Source: three-view drawing plus pictorial views. Frame: mm from the lowest corner of the part. A direction names the side the tool comes from. Give positions to 0.01 mm unless a question says otherwise; leave off trailing zeros. Loops run counter-clockwise (first coordinate to the right, second up) from the corner with the lowest first, then second, coordinate; pieces in that order, holes last. Notation, with made-up numbers: M 23,52.25 L 40,52.25 A17 cw 40,66.25 Z; hole C -16,72.25 d1. An arc over 180 degrees is marked long. Write item = value, one per line.
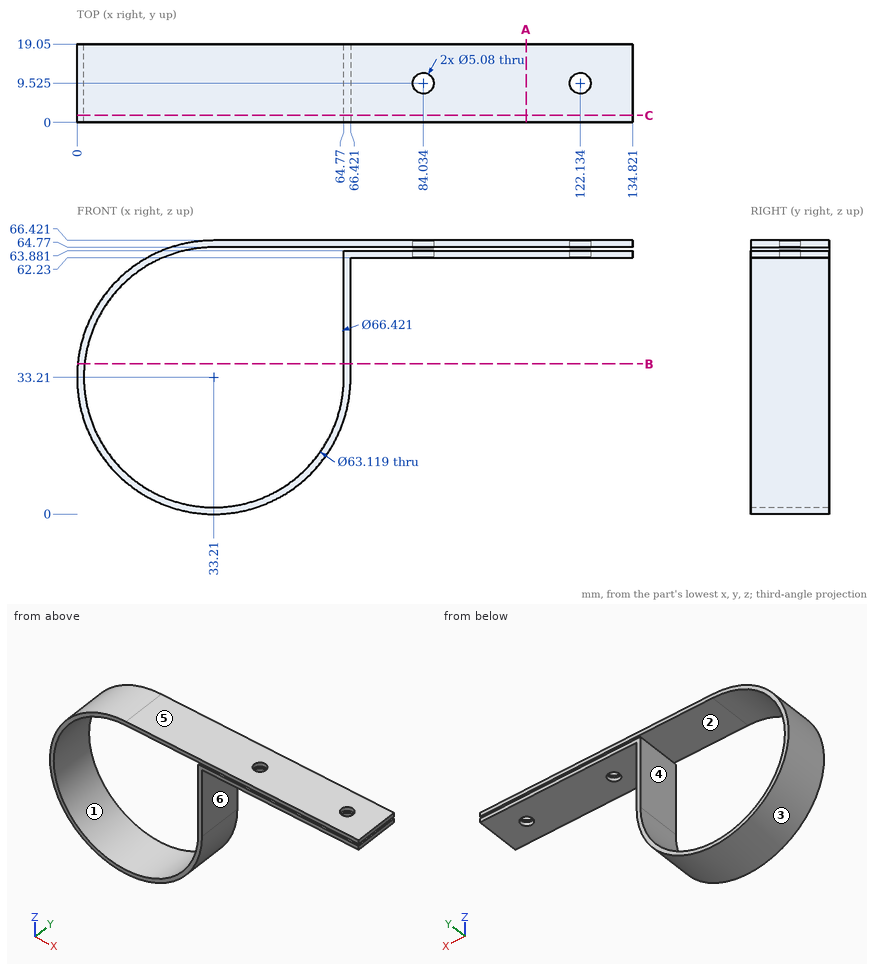
1. Pull-direction query (X, two-part tool) for the marked faces 1, 2 and 3; classes: +X half, -X half, draft (parallel to the pull), parting line (faces both ways), or undercut.
Derived:
face_1 = undercut
face_2 = draft
face_3 = parting line
2. Material intervals for probe 1 along Z at (x, y) = (34, 15.75); probe 2 along Z at (x, y) = (101.5, 1); probe 3 along X at (y, z) = (17, 32.5), sorted ascending. Write a range as from..to.
Derived:
probe_1 = 0.01..1.66, 64.77..66.42
probe_2 = 62.23..63.88, 64.77..66.42
probe_3 = 0.01..1.66, 64.76..66.41
3. Cut plane B-B, the plane z = 36.5. Return the cut outline in (x, y).
Derived:
outline = M 0.16,0 L 1.82,0 L 1.82,19.05 L 0.16,19.05 Z; M 64.77,0 L 66.42,0 L 66.42,19.05 L 64.77,19.05 Z
4. Reachability of the marked faces 4, 5 and 6 from +Z, -Z, +X, -X, +Y, -Y: full face, straight path, thin tool, end or side. Return the list, or none.
Derived:
face_4 = +Y, -Y
face_5 = +Z, +X, -X, +Y, -Y
face_6 = -Z, +X, +Y, -Y
5. First-contact query: pin 1 Ø6.5 at (x, y) = (122.13, 9.52) entering from -Z; pin 2 Ø1.5 at (x, y) = (30.5, 6) entering from -Z; pin 3 Ø2 at (y, z) = (9, 11) entering from -X (1 decimal). Flat tips, straight axial feed; report the tip coordinate or a pass-through.
Derived:
pin_1 = 62.23
pin_2 = 0.06
pin_3 = 7.7
6. Cut plane C-C, the plane y = 1.75. Return the cut outline in (x, z).
Derived:
outline = M 33.22,64.77 L 134.82,64.77 L 134.82,66.42 L 33.22,66.42 A33.21 ccw long 66.42,33.21 L 66.42,62.23 L 134.82,62.23 L 134.82,63.88 L 64.77,63.88 L 64.77,33.21 A31.56 cw long Z
7. Cut plane A-A, the plane x = 109. Return the cut outline in (y, z).
Derived:
outline = M 0,62.23 L 19.05,62.23 L 19.05,63.88 L 0,63.88 Z; M 0,64.77 L 19.05,64.77 L 19.05,66.42 L 0,66.42 Z
